```python
from build123d import *

# Parameters (mm, degrees)
F0_R     = 2.5
F1_DEPTH = 10


with BuildPart() as f1:
    # F0 (on Front) → F1 (new body)
    with BuildSketch(Plane.XZ):
        with BuildLine():
            ThreePointArc((39.68627, -5), (39.92149, -2.504917), (40, 0))
            ThreePointArc((40, 0), (39.92149, 2.504917), (39.68627, 5))
            ThreePointArc((39.68627, 5), (28.284271, 28.284271), (5, 39.68627))
            ThreePointArc((5, 39.68627), (0, 40), (-5, 39.68627))
            ThreePointArc((-5, 39.68627), (-28.284271, 28.284271), (-39.68627, 5))
            ThreePointArc((-39.68627, 5), (-40, 0), (-39.68627, -5))
            ThreePointArc((-39.68627, -5), (-28.284271, -28.284271), (-5, -39.68627))
            ThreePointArc((-5, -39.68627), (0, -40), (5, -39.68627))
            ThreePointArc((5, -39.68627), (28.284271, -28.284271), (39.68627, -5))
        make_face()
        with BuildLine():
            ThreePointArc((-5, -30.594117), (-21.92031, -21.92031), (-30.594117, -5))
            Line((-30.594117, -5), (-5.59017, -5))
            ThreePointArc((-5.59017, -5), (-5.303301, -5.303301), (-5, -5.59017))
            Line((-5, -5.59017), (-5, -30.594117))
        make_face(mode=Mode.SUBTRACT)
        with BuildLine():
            Line((5, -30.594117), (5, -5.59017))
            ThreePointArc((5, -5.59017), (5.303301, -5.303301), (5.59017, -5))
            Line((5.59017, -5), (30.594117, -5))
            ThreePointArc((30.594117, -5), (21.92031, -21.92031), (5, -30.594117))
        make_face(mode=Mode.SUBTRACT)
        with BuildLine():
            Line((-5, 30.594117), (-5, 5.59017))
            ThreePointArc((-5, 5.59017), (-5.303301, 5.303301), (-5.59017, 5))
            Line((-5.59017, 5), (-30.594117, 5))
            ThreePointArc((-30.594117, 5), (-21.92031, 21.92031), (-5, 30.594117))
        make_face(mode=Mode.SUBTRACT)
        Circle(F0_R, mode=Mode.SUBTRACT)
        with BuildLine():
            Line((30.594117, 5), (5.59017, 5))
            ThreePointArc((5.59017, 5), (5.303301, 5.303301), (5, 5.59017))
            Line((5, 5.59017), (5, 30.594117))
            ThreePointArc((5, 30.594117), (21.92031, 21.92031), (30.594117, 5))
        make_face(mode=Mode.SUBTRACT)
    extrude(amount=F1_DEPTH)


solid = f1.part
```
Design review of the part built by this model. Coordinates are the model's own, in mm. A direction names the side the tool comes from. Coordinates: 2 decimals unless noted, no trailing zeros. Loops run counter-clockwise (first coordinate to the right, second up) from the corner with the lowest first, then second, coordinate; pieces in that order, holes last.
Q1. We need section A-A on y = -4. State the section outline as (x, z) points.
Reported:
outline: (-39.69, -5) arc R40 ccw to (-5, -39.69) arc R40 ccw to (5, -39.69) arc R40 ccw to (39.69, -5) arc R40 ccw to (40, 0) arc R40 ccw to (39.69, 5) arc R40 ccw to (5, 39.69) arc R40 ccw to (-5, 39.69) arc R40 ccw to (-39.69, 5) arc R40 ccw to start; hole (-30.59, -5) arc R31 ccw to (-5, -30.59) - (-5, -5.59) arc R7.5 cw to (-5.59, -5) - close; hole (-30.59, 5) - (-5.59, 5) arc R7.5 cw to (-5, 5.59) - (-5, 30.59) arc R31 ccw to start; hole circle Ø5 at (0, 0); hole (5, -30.59) arc R31 ccw to (30.59, -5) - (5.59, -5) arc R7.5 cw to (5, -5.59) - close; hole (5, 5.59) arc R7.5 cw to (5.59, 5) - (30.59, 5) arc R31 ccw to (5, 30.59) - close
Q2. To check wall thickness, follow line 1 (Z direction, x = 0, y = -5.25); line 2 (Z direction, x = -23, y = -4.5); line 3 (Z direction, x = 16.5, y = -3). State the ranges of each line that lie inside material, in increasing order.
Reported:
line 1: z = -40 to -2.5, 2.5 to 40
line 2: z = -32.73 to -20.78, -5 to 5, 20.78 to 32.73
line 3: z = -36.44 to -26.24, -5 to 5, 26.24 to 36.44
Q3. Tool access review of faces 1 (the face through (-1, -10, -8)), 2 (the face through (5, -5, -18)): name each direction out of +Z, -Z, +X, -X, +Y, -Y from which nothing blocks a thin tool from reaching the whole face with its end or side.
Reported:
face 1: +Z, -Z, +X, -X, -Y
face 2: +Y, -Y
Q4. For pin 1 (5 mm diameter, centred on x = -19.5, y = -4.5, fed in from -Z); pin 2 (3 mm diameter, centred on y = -5.5, z = -17, fed in from -X); pin 3 (5 mm diameter, centred on x = 13.5, y = -6, fed in from -Z), all flat-tipped, find the tip position at first contact; note any pin that passes through.
Reported:
pin 1: stops at z = -36.21
pin 2: stops at x = -36.87
pin 3: stops at z = -38.46
Q5. We need section B-B on z = -23. State the section outline as (x, y) points.
Reported:
outline: (-32.73, -10) - (-20.78, -10) - (-20.78, 0) - (-32.73, 0) - close; (-5, -10) - (5, -10) - (5, 0) - (-5, 0) - close; (20.78, -10) - (32.73, -10) - (32.73, 0) - (20.78, 0) - close
Q6. The part is to be moulded in two halves that separate along X. For faces 3 (the face through (-0.54, -4.93, -2.44)), 4 (the face through (28.022, -4.93, -28.544)), 5 (the face through (0, -5, 40)), say which applies: +X half, -X half, draft (parallel to the pull), parting line (faces both ways), or undercut.
Reported:
face 3: undercut
face 4: +X half
face 5: parting line
Q7. We need section D-D on x = 0. State the section outline as (y, z) points, and give its area (3 significant figures).
Reported:
outline: (-10, -40) - (0, -40) - (0, -2.5) - (-10, -2.5) - close; (-10, 2.5) - (0, 2.5) - (0, 40) - (-10, 40) - close
area: 750 mm2
Q8. We need section C-C on x = 18.5. State the section outline as (y, z) points, and give its area (3 significant figures).
Reported:
outline: (-10, -35.46) - (0, -35.46) - (0, -24.87) - (-10, -24.87) - close; (-10, -5) - (0, -5) - (0, 5) - (-10, 5) - close; (-10, 24.87) - (0, 24.87) - (0, 35.46) - (-10, 35.46) - close
area: 312 mm2
